Geometry check sheet. Reference: the model listing, model coordinates, mm. Round coordinates to 2 decimals unless told otherwise and drop trailing zeros. Loops run counter-clockwise (first coordinate to the right, second up) from the corner with the lowest first, then second, coordinate; pieces in that order, holes last.
```python
from build123d import *

# Parameters (mm, degrees)
PAD_DEPTH     = 16
SKETCH001_R   = 15
SKETCH001_R_2 = 10
POCKET_DEPTH  = 16.001


with BuildPart() as part:
    # Sketch → Pad (new body)
    with BuildSketch(Plane.XY):
        Polygon((0, 500), (150, 500), (150, 0), (0, 0), (0, 250), align=None)
    extrude(amount=PAD_DEPTH)

    # Sketch001 (on Face7 of Pad) → Pocket (cut, through all)
    with BuildSketch(Plane.XY.offset(16)):
        with Locations((31.579084, 67.777323)):
            Circle(SKETCH001_R)
        with Locations((50.054292, 99.777323)):
            Circle(SKETCH001_R)
        with Locations((68.529501, 131.777323)):
            Circle(SKETCH001_R)
        with Locations((50.054292, 163.777323)):
            Circle(SKETCH001_R)
        with Locations((71, 246.635039)):
            Circle(SKETCH001_R_2)
        with Locations((68.529501, 67.777323)):
            Circle(SKETCH001_R)
        with Locations((88.15941, 101.777323)):
            Circle(SKETCH001_R)
        with Locations((88.15941, 163.777323)):
            Circle(SKETCH001_R)
        with Locations((53.441466, 300.257294)):
            Circle(SKETCH001_R)
        with Locations((71.916674, 332.257294)):
            Circle(SKETCH001_R)
        with Locations((90.391883, 364.257294)):
            Circle(SKETCH001_R)
        with Locations((71.916674, 396.257294)):
            Circle(SKETCH001_R)
        with Locations((71, 458)):
            Circle(SKETCH001_R_2)
        with Locations((90.391883, 300.257294)):
            Circle(SKETCH001_R)
        with Locations((110.021792, 334.257294)):
            Circle(SKETCH001_R)
        with Locations((110.021792, 396.257294)):
            Circle(SKETCH001_R)
    extrude(amount=-POCKET_DEPTH, mode=Mode.SUBTRACT)


solid = part.part
```
1) Scan lines: line 1 along X through (y, z) = (133, 12.25); line 2 along Y through (x, z) = (112, 3); line 3 along X through (y, z) = (345.5, 11.5). Record each from-to range of solid material in increasing order.
Report:
line 1: x = 0 to 53.58, 83.48 to 150
line 2: y = 0 to 319.39, 349.13 to 381.39, 411.13 to 500
line 3: x = 0 to 64.87, 78.96 to 100.09, 119.95 to 150
2) Sectioned sample at B-B, the plane z = 12.75. State how many separate pieces and enclosed holes the cut face has, then the cut area to 3 significant figures.
Report:
separate pieces: 1
enclosed holes: 16
area: 64,500 mm2
3) Sectioned sample at A-A, the plane y = 458. Record the cut outline in (x, z), then the cut area to 3 significant figures.
Report:
outline: (0, 0) - (61, 0) - (61, 16) - (0, 16) - close; (81, 0) - (150, 0) - (150, 16) - (81, 16) - close
area: 2,080 mm2
4) Mould release check, pull along X, two halves, no side actions. Record for faces 1 (the face through (0, 253, 8)), 2 (the face through (150, 253, 8)), 3 (the face through (66.58, 146.65, 8.11)), 4 (the face through (93, 254, 16)): +X half, -X half, draft (parallel to the pull), parting line (faces both ways), or undercut.
Report:
face 1: -X half
face 2: +X half
face 3: undercut
face 4: draft
